CAD build for the part. Positions are in the model's coordinates, mm. Face numbers are marked on the shaded views. A direction names the side the tool comes from. Round coordinates to 2 decimals unless told otherwise and drop trailing zeros. Loops run counter-clockwise (first coordinate to the right, second up) from the corner with the lowest first, then second, coordinate; pieces in that order, holes last.
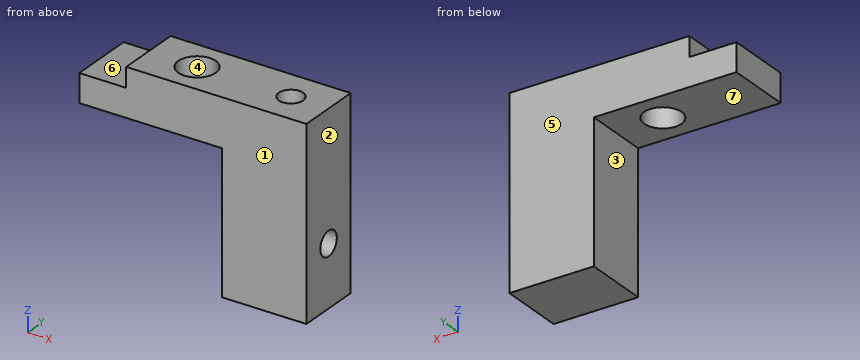
from build123d import *

# Parameters (mm, degrees)
PAD025_DEPTH             = 3.5
PAD025_DEPTH_BACK        = 3.5
SKETCH047_R              = 2
SKETCH047_R_2            = 1.3
POCKET_DEPTH             = 8
SKETCH049_R              = 1.3
POCKET001_DEPTH          = 8
CLONE010_PLACEMENT_ANGLE = 180


with BuildPart() as part:
    # Sketch → Pad025 (new body, two sides)
    with BuildSketch(Plane.XZ) as pad025_sk:
        Polygon((-58.82, -4.5), (-58.82, -6.6), (-53.82, -6.6), (-53.82, -9.6), (-69, -9.6), (-69, -24.5), (-78, -24.5), (-78, -4.5), align=None)
    extrude(amount=PAD025_DEPTH)
    extrude(pad025_sk.sketch, amount=-PAD025_DEPTH_BACK)

    # Sketch047 → Pocket (cut)
    with BuildSketch(Plane(origin=(0, 0, -9.6), x_dir=(1, 0, 0), z_dir=(0, 0, -1))):
        with Locations((-64, 0)):
            Circle(SKETCH047_R)
        with Locations((-74, 0)):
            Circle(SKETCH047_R_2)
    extrude(amount=-POCKET_DEPTH, mode=Mode.SUBTRACT)

    # Sketch049 → Pocket001 (cut)
    with BuildSketch(Plane(origin=(-78, 0, 0), x_dir=(0, 0, -1), z_dir=(-1, 0, 0))):
        with Locations((18, 0)):
            Circle(SKETCH049_R)
    extrude(amount=-POCKET001_DEPTH, mode=Mode.SUBTRACT)


with BuildPart() as part_1:
    # Clone010 placement: moved
    add(part.part.moved(Location((0, -27, 0))).rotate(Axis((0, -27, 0), (0, 0, 1)), CLONE010_PLACEMENT_ANGLE))


solid = part_1.part
Item 1: Cut at A-A (x = 64). List the corners of the cut face in (y, z).
Verdict:
outline: (-30.5, -9.6) - (-29, -9.6) - (-29, -4.5) - (-30.5, -4.5) - close; (-25, -9.6) - (-23.5, -9.6) - (-23.5, -4.5) - (-25, -4.5) - close
Item 2: Wall check: L1, parallel to X at y = -27, z = -5.65; L2, parallel to X at y = -27, z = -6.7; L3, parallel to Y at x = 74, z = -6.1. Give the ranges that are in metal, low to high.
Verdict:
L1: x = 58.82 to 62, 66 to 72.7, 75.3 to 78
L2: x = 53.82 to 62, 66 to 72.7, 75.3 to 78
L3: y = -30.5 to -28.3, -25.7 to -23.5
Item 3: Cut at C-C (z = -18). List the corners of the cut face in (x, y).
Verdict:
outline: (69, -30.5) - (78, -30.5) - (78, -28.3) - (70, -28.3) - (70, -25.7) - (78, -25.7) - (78, -23.5) - (69, -23.5) - close
Item 4: 3-axis set-ups, long thin cutter, end or side, ignore diameter. For the marked faces 5, 6 and 7: which of +Z, -Z, +X, -X, +Y, -Y reach the whole face in a straight line?
Verdict:
face 5: +Z, -Z, +X, -X, +Y
face 6: +Z, -X, +Y, -Y
face 7: -Z, -X, +Y, -Y
Item 5: Cut at D-D (x = 74). List the corners of the cut face in (y, z), plus the area to 3 significant figures.
Verdict:
outline: (-30.5, -24.5) - (-23.5, -24.5) - (-23.5, -4.5) - (-25.7, -4.5) - (-25.7, -9.6) - (-28.3, -9.6) - (-28.3, -4.5) - (-30.5, -4.5) - close; hole circle Ø2.6 at (-27, -18)
area: 121 mm2
Item 6: Mould opens along X. For the marked faces 1, 2, 3 and 4 say: released by +X, released by -X, zero draft, split by the parting line, or undercut.
Verdict:
face 1: zero draft
face 2: released by +X
face 3: released by -X
face 4: undercut
Item 7: Cut at B-B (y = -27.75). List the corners of the cut face in (x, z).
Verdict:
outline: (53.82, -9.6) - (62.15, -9.6) - (62.15, -4.5) - (58.82, -4.5) - (58.82, -6.6) - (53.82, -6.6) - close; (65.85, -9.6) - (69, -9.6) - (69, -24.5) - (78, -24.5) - (78, -19.06) - (70, -19.06) - (70, -16.94) - (78, -16.94) - (78, -4.5) - (75.06, -4.5) - (75.06, -9.6) - (72.94, -9.6) - (72.94, -4.5) - (65.85, -4.5) - close
Item 8: Flat gauge pins, fed straight in: P1, Ø1.5, axis at y = -28.5, z = -11.5, coming from the -X side; P2, Ø3.5, axis at x = 65, y = -26.5, coming from the -Z side; P3, Ø1.7, axis at y = -26, z = -5, coming from the -X side. Where does each tip first touch, or does it go through?
Verdict:
P1: stops at x = 69
P2: stops at z = -9.6
P3: stops at x = 58.82
